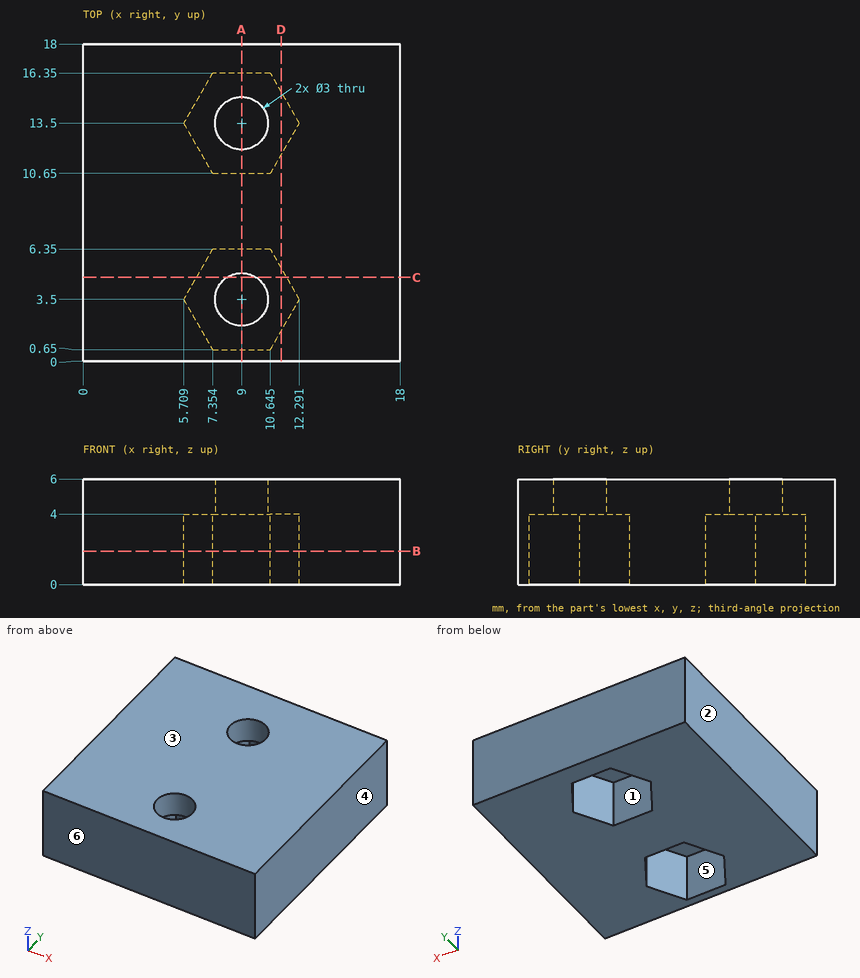
Could you check a few things on this drawing? It's one solid part, dimensions in mm from its lowest x, y, z. A direction names the side the tool comes from. Round coordinates to 2 decimals unless told otherwise and drop trailing zeros. Order: outer loops, then holes, each group sorted by start corner. A loop starts at its lowest first (then second) coordinate and runs counter-clockwise, first axis right, second up.
(1) If we mould it in two halves opening along X, with no side actions, what happens to the marked faces 1, 2, 3 and 4? For each: released by +X, released by -X, zero draft, split by the parting line, or undercut.
Response values:
face 1: undercut
face 2: released by -X
face 3: zero draft
face 4: released by +X
(2) Imagine slicing it at C-C (y = 4.75). Write out the boundary of the cut face in (x, z).
Response values:
outline: (0, 0) - (6.43, 0) - (6.43, 4) - (8.17, 4) - (8.17, 6) - (0, 6) - close; (9.83, 4) - (11.57, 4) - (11.57, 0) - (18, 0) - (18, 6) - (9.83, 6) - close
(3) Imagine slicing it at A-A (x = 9). Write out the boundary of the cut face in (y, z).
Response values:
outline: (0, 0) - (0.65, 0) - (0.65, 4) - (2, 4) - (2, 6) - (0, 6) - close; (5, 4) - (6.35, 4) - (6.35, 0) - (10.65, 0) - (10.65, 4) - (12, 4) - (12, 6) - (5, 6) - close; (15, 4) - (16.35, 4) - (16.35, 0) - (18, 0) - (18, 6) - (15, 6) - close
(4) Imagine slicing it at D-D (x = 11.25). Write out the boundary of the cut face in (y, z).
Response values:
outline: (0, 0) - (1.7, 0) - (1.7, 4) - (5.3, 4) - (5.3, 0) - (11.7, 0) - (11.7, 4) - (15.3, 4) - (15.3, 0) - (18, 0) - (18, 6) - (0, 6) - close
(5) Which directions (+Z, -Z, +X, -X, +Y, -Y) give clear straight access to the entire face, cutting with the end or side of a thin tool? Please do the marked faces 5 and 6.
Response values:
face 5: -Z
face 6: +Z, -Z, +X, -X, -Y
(6) I'm going to push a flat-ended pin straight in: pin 1 (3.5 mm diameter, centred on x = 9, y = 3.5, fed in from -Z). Where does the tip first touch, or does it pass through?
Response values:
pin 1: stops at z = 4
(7) Please list where these lines run through material, in increasing order: line 1 along Y through (x, z) = (9, 4.65); line 2 along Y through (x, z) = (8.5, 1.3); line 3 along X through (y, z) = (3.5, 4.75).
Response values:
line 1: y = 0 to 2, 5 to 12, 15 to 18
line 2: y = 0 to 0.65, 6.35 to 10.65, 16.35 to 18
line 3: x = 0 to 7.5, 10.5 to 18
(8) Imagine slicing it at B-B (z = 1.9). Count the separate pieces of the cut face and the enclosed holes in it, plus the area to 3 significant figures.
Response values:
separate pieces: 1
enclosed holes: 2
area: 268 mm2
